Geometry: final body of the model. Coordinates: model frame, mm. A direction names the side the tool comes from. Give positions to 0.01 mm unless a question says otherwise; leave off trailing zeros. Write each loop counter-clockwise with the first axis right and the second up, starting at its lowest first coordinate (ties: lowest second). Pieces come first, ordered by that corner, then holes. Notation, with made-up numbers: M 1,66 L 11,66 A18 ccw 11,70 Z; hole C 30,-11.5 d10. An arc over 180 degrees is marked long. Use a Markdown table: item, result. Add a question column.
(1) Reachability of faces 3 (the flat face through (38, 51.978, 6)), 4 (the flat face through (42.799, 50, 1)), 5 (the flat face through (26, 2.54, 5)) from +Z, -Z, +X, -X, +Y, -Y: full face, straight path, thin tool, end or side. Return the list, or none.
(2) Draft query along X for faces 1 (the flat face through (26, 50, -3.238)), 2 (the flat face through (0, 33, 3)). Return one class per face: released by +X, released by -X, zero draft, split by the parting line, or undercut.
(3) Cut plane B-B (z = 1.5). Output: boundary loops of the cut face in (x, y).
(4) Material intervals for L1, parallel to Y at x = 42.5, z = 4; L2, parallel to X at y = 24, z = 4.75; L3, parallel to Y at x = 38, z = -3.5, sorted ascending.
(5) Cut plane A-A (y = 25). Output: boundary loops of the cut face in (x, z), plus the area to 3 significant figures.
(6) Cut plane D-D (y = 8). Output: boundary loops of the cut face in (x, z), plus the area to 3 significant figures.
(7) Pin query (flat end, axial travel): pin 1 Ø8 at (x, y) = (44, 15.5) entering from -Z; pin 2 Ø2 at (x, y) = (7.5, 12) entering from +Z; pin 3 Ø3 at (x, z) = (39.5, 1) entering from +Y. Return the tip coordinate at first contact, or that it passes through.
(8) Cut plane C-C (x = 36). Output: boundary loops of the cut face in (y, z), plus the area to 3 significant figures.
```python
from build123d import *

# Parameters (mm, degrees)
SKETCH1_W                       = 52.07
SKETCH1_H                       = 26.416
ULTRASONIC_HOLDER_EXTRUDE_DEPTH = 7.62
ULTRASONIC_CUTOUT_T             = -2.54
ULTRASONIC_WIRE_HOLE_DEPTH      = 6.35
ULTRASONIC_WIRE_HOLE_DEPTH_BACK = 12.7
ULTRASONIC_WIRE_HOLE_START      = -26.416
SKETCH2_W                       = 13.97
SKETCH2_H                       = 7.62
SKETCH7_W                       = 12.7
SKETCH7_H                       = 9.56038728
SERVO_HOLDER_DEPTH              = 52.07
SKETCH10_W                      = 9.144
SKETCH10_H                      = 7.62
CONNECTOR_DEPTH                 = 20.32
SERVO_CUTOUT_DEPTH              = 7.62
SERVO_SECURER_CUT_DEPTH         = 76.909973478
SERVO_SECURER_CUT_DEPTH_BACK    = 76.909973478
SKETCH15_W                      = 8.215827997
SKETCH15_H                      = 2.032


with BuildPart() as part:
    # Sketch1 → Ultrasonic Holder Extrude (new body)
    with BuildSketch(Plane.XY):
        with Locations((26.035, 13.208)):
            Rectangle(SKETCH1_W, SKETCH1_H)
    extrude(amount=ULTRASONIC_HOLDER_EXTRUDE_DEPTH)

    # Ultrasonic Cutout
    ultrasonic_cutout_openings = [part.faces().sort_by_distance(p)[0] for p in [
        (26.035, 13.208, 7.62),
    ]]
    offset(amount=ULTRASONIC_CUTOUT_T, openings=ultrasonic_cutout_openings, kind=Kind.INTERSECTION)

    # Sketch2 → Ultrasonic Wire Hole (cut, two sides: drawn at the far end of the back side and taken through both)
    with BuildSketch(Plane.XZ.offset(ULTRASONIC_WIRE_HOLE_START - ULTRASONIC_WIRE_HOLE_DEPTH_BACK)):
        with Locations((26.035, 3.81)):
            Rectangle(SKETCH2_W, SKETCH2_H)
    extrude(amount=ULTRASONIC_WIRE_HOLE_DEPTH + ULTRASONIC_WIRE_HOLE_DEPTH_BACK, mode=Mode.SUBTRACT)



with BuildPart() as body_2:
    # Sketch7 → Servo Holder (new, through all)
    with BuildSketch(Plane.ZY):
        with Locations((1.27, 48.97619364)):
            Rectangle(SKETCH7_W, SKETCH7_H)
    extrude(amount=-SERVO_HOLDER_DEPTH)


with BuildPart() as part_1:
    add(part.part)

    add(body_2.part)  # Connector merges body 2
    # Sketch10 → Connector (add)
    with BuildSketch(Plane.XZ.offset(-44.196)):
        with Locations((4.572, 3.81)):
            Rectangle(SKETCH10_W, SKETCH10_H)
        with Locations((47.498, 3.81)):
            Rectangle(SKETCH10_W, SKETCH10_H)
    extrude(amount=CONNECTOR_DEPTH)

    # Sketch14 → Servo Cutout (cut)
    with BuildSketch(Plane.ZX.offset(53.75638728)):
        Polygon((-1.11125, 42.799), (3.65125, 42.799), (5.7785, 28.0162), (5.7785, 24.0538), (3.65125, 9.271), (-1.11125, 9.271), (-3.2385, 24.0538), (-3.2385, 28.0162), align=None)
    extrude(amount=-SERVO_CUTOUT_DEPTH, mode=Mode.SUBTRACT)

    # Sketch15 → Servo Securer Cut (cut, two sides: drawn at the far end of the back side and taken through both)
    with BuildSketch(Plane.XY.offset(7.62).offset(-SERVO_SECURER_CUT_DEPTH_BACK)):
        with Locations((14.288933515, 50.96238728)):
            Rectangle(SKETCH15_W, SKETCH15_H)
        with Locations((37.802086002, 50.96238728)):
            Rectangle(SKETCH15_W, SKETCH15_H)
    extrude(amount=SERVO_SECURER_CUT_DEPTH + SERVO_SECURER_CUT_DEPTH_BACK, mode=Mode.SUBTRACT)


solid = part_1.part
```
Answer list:
| question | item | result |
|---|---|---|
| 1 | face 3 | +Z, -Z |
| 1 | face 4 | +Y |
| 1 | face 5 | +Z |
| 2 | face 1 | undercut |
| 2 | face 2 | released by -X |
| 3 | outline | M 0,0 L 52.07,0 L 52.07,53.76 L 42.8,53.76 L 42.8,46.14 L 9.27,46.14 L 9.27,53.76 L 0,53.76 Z; hole M 9.14,26.42 L 19.05,26.42 L 19.05,20.07 L 33.02,20.07 L 33.02,26.42 L 42.93,26.42 L 42.93,44.2 L 9.14,44.2 Z |
| 4 | L1 | 0 to 2.54, 23.88 to 26.42, 44.2 to 53.76 |
| 4 | L2 | 0 to 19.05, 33.02 to 52.07 |
| 4 | L3 | 44.2 to 49.95, 51.98 to 53.76 |
| 5 | outline | M 0,0 L 19.05,0 L 19.05,7.62 L 0,7.62 Z; M 33.02,0 L 52.07,0 L 52.07,7.62 L 33.02,7.62 Z |
| 5 | area | 290 mm² |
| 6 | outline | M 0,0 L 52.07,0 L 52.07,7.62 L 49.53,7.62 L 49.53,2.54 L 2.54,2.54 L 2.54,7.62 L 0,7.62 Z |
| 6 | area | 158 mm² |
| 7 | pin 1 | z = 0 |
| 7 | pin 2 | z = 2.54 |
| 7 | pin 3 | y = 46.14 |
| 8 | outline | M 0,0 L 26.42,0 L 26.42,7.62 L 23.88,7.62 L 23.88,2.54 L 2.54,2.54 L 2.54,7.62 L 0,7.62 Z; M 44.2,-5.08 L 49.95,-5.08 L 49.95,-2.09 L 46.14,-2.09 L 46.14,4.63 L 49.95,4.63 L 49.95,7.62 L 44.2,7.62 Z; M 51.98,-5.08 L 53.76,-5.08 L 53.76,-2.09 L 51.98,-2.09 Z; M 51.98,4.63 L 53.76,4.63 L 53.76,7.62 L 51.98,7.62 Z |
| 8 | area | 151 mm² |
